from build123d import *

# Parameters (mm, degrees)
EXTRUDE_1_DEPTH     = 2
SKETCH_2_W          = 50
SKETCH_2_H          = 27
EXTRUDE_2_DEPTH     = 10
SKETCH_3_R          = 3
CUT_EXTRUDE_1_DEPTH = 13
SKETCH_5_W          = 47
SKETCH_5_H          = 1.6
CUT_EXTRUDE_2_DEPTH = 1.6
SKETCH_6_W          = 4
SKETCH_6_H          = 10
CUT_EXTRUDE_3_DEPTH = 7
SKETCH_7_W          = 80
SKETCH_7_H          = 14.002207555
CUT_EXTRUDE_4_DEPTH = 10
CUT_EXTRUDE_5_REACH = 14


with BuildPart() as part:
    # 草图1 → 凸台-拉伸1 (new body)
    with BuildSketch(Plane.XY):
        with BuildLine():
            Line((-46, 22.841953517), (-46, -22.841953517))
            Line((-46, -22.841953517), (-51, -31.502207555))
            Line((-51, -31.502207555), (-51, -39.502207555))
            ThreePointArc((-51, -39.502207555), (-46, -44.502207555), (-41, -39.502207555))
            Line((-41, -39.502207555), (-41, -31.502207555))
            Line((-41, -31.502207555), (36, -31.502207555))
            Line((36, -31.502207555), (36, -39.502207555))
            ThreePointArc((36, -39.502207555), (41, -44.502207555), (46, -39.502207555))
            Line((46, -39.502207555), (46, 39.502207555))
            ThreePointArc((46, 39.502207555), (41, 44.502207555), (36, 39.502207555))
            Line((36, 39.502207555), (36, 31.502207555))
            Line((36, 31.502207555), (-41, 31.502207555))
            Line((-41, 31.502207555), (-41, 39.502207555))
            ThreePointArc((-41, 39.502207555), (-46, 44.502207555), (-51, 39.502207555))
            Line((-51, 39.502207555), (-51, 31.502207555))
            Line((-51, 31.502207555), (-46, 22.841953517))
        make_face()
    extrude(amount=EXTRUDE_1_DEPTH)

    # 草图2 → 凸台-拉伸2 (add)
    with BuildSketch(Plane(origin=(0, 0, 0), x_dir=(-1, 0, 0), z_dir=(0, 0, -1))):
        with BuildLine():
            Line((46, -22.841953517), (46, 22.841953517))
            Line((46, 22.841953517), (51, 31.502207555))
            Line((51, 31.502207555), (51, 39.502207555))
            ThreePointArc((51, 39.502207555), (46, 44.502207555), (41, 39.502207555))
            Line((41, 39.502207555), (41, 31.502207555))
            Line((41, 31.502207555), (-36, 31.502207555))
            Line((-36, 31.502207555), (-36, 39.502207555))
            ThreePointArc((-36, 39.502207555), (-41, 44.502207555), (-46, 39.502207555))
            Line((-46, 39.502207555), (-46, -39.502207555))
            ThreePointArc((-46, -39.502207555), (-41, -44.502207555), (-36, -39.502207555))
            Line((-36, -39.502207555), (-36, -31.502207555))
            Line((-36, -31.502207555), (41, -31.502207555))
            Line((41, -31.502207555), (41, -39.502207555))
            ThreePointArc((41, -39.502207555), (46, -44.502207555), (51, -39.502207555))
            Line((51, -39.502207555), (51, -31.502207555))
            Line((51, -31.502207555), (46, -22.841953517))
        make_face()
        with Locations((-15, 0)):
            Rectangle(SKETCH_2_W, SKETCH_2_H, mode=Mode.SUBTRACT)
    extrude(amount=EXTRUDE_2_DEPTH)

    # 草图3 → 切除-拉伸1 (cut, through all)
    with BuildSketch(Plane(origin=(0, 0, -10), x_dir=(-1, 0, 0), z_dir=(0, 0, -1))):
        with Locations((-41, 39.502207555)):
            Circle(SKETCH_3_R)
        with Locations((46, -39.502207555)):
            Circle(SKETCH_3_R)
        with Locations((46, 39.502207555)):
            Circle(SKETCH_3_R)
        with Locations((-41, -39.502207555)):
            Circle(SKETCH_3_R)
    extrude(amount=-CUT_EXTRUDE_1_DEPTH, mode=Mode.SUBTRACT)

    # 草图5 → 切除-拉伸2 (cut)
    with BuildSketch(Plane(origin=(0, 0, 0), x_dir=(-1, 0, 0), z_dir=(0, 0, -1))):
        with Locations((-15.3, 10.95)):
            Rectangle(SKETCH_5_W, SKETCH_5_H)
        with Locations((-15.3, -10.95)):
            Rectangle(SKETCH_5_W, SKETCH_5_H)
    extrude(amount=-CUT_EXTRUDE_2_DEPTH, mode=Mode.SUBTRACT)

    # 草图6 → 切除-拉伸3 (cut, through all)
    with BuildSketch(Plane.ZY.offset(-40)):
        with Locations((-8, 0.5)):
            Rectangle(SKETCH_6_W, SKETCH_6_H)
    extrude(amount=-CUT_EXTRUDE_3_DEPTH, mode=Mode.SUBTRACT)

    # 草图7 → 切除-拉伸4 (cut)
    with BuildSketch(Plane(origin=(0, 0, -10), x_dir=(-1, 0, 0), z_dir=(0, 0, -1))):
        with Locations((4, -22.501103778)):
            Rectangle(SKETCH_7_W, SKETCH_7_H)
        Polygon((12, -15.5), (44, -15.5), (44, 29.502207555), (-36, 29.502207555), (-36, 15.5), (12, 15.5), align=None)
    extrude(amount=-CUT_EXTRUDE_4_DEPTH, mode=Mode.SUBTRACT)

    # 草图9 → 切除-拉伸5 (cut, up to next)
    with BuildSketch(Plane(origin=(0, 0, -10), x_dir=(-1, 0, 0), z_dir=(0, 0, -1)), mode=Mode.PRIVATE) as cut_extrude_5_sk1:
        Polygon((-46, -35.502207555), (-41.2, -28.502207555), (-41.2, 28.502207555), (-46, 35.502207555), align=None)
    cut_extrude_5_tool1 = extrude(cut_extrude_5_sk1.sketch, amount=-CUT_EXTRUDE_5_REACH, mode=Mode.PRIVATE) & part.part
    add(cut_extrude_5_tool1.solids().sort_by_distance((43.687494, 0, -10))[0], mode=Mode.SUBTRACT)


solid = part.part
Build history of the part. All positions in model axes, mm. A direction names the side the tool comes from. Round coordinates to 2 decimals unless told otherwise and drop trailing zeros. Loops run counter-clockwise (first coordinate to the right, second up) from the corner with the lowest first, then second, coordinate; pieces in that order, holes last. Notation, with made-up numbers: (83, 31) -> (139, 31) arc R32 ccw to (139, 58) -> close; hole circle Ø11 at (13, 4.25). An arc over 180 degrees is marked (long way). Use CSV: the item, a comma, the result in double quotes. Start each with the question number.
Q1. Flat gauge pins, fed straight in: pin 1 Ø3 at (x, z) = (13.5, -6) entering from -Y; pin 2 Ø2 at (x, y) = (28, 0) entering from -Z; pin 3 Ø5 at (y, z) = (-0.5, -6) entering from +X; pin 4 Ø5 at (x, y) = (41, 39.5) entering from +Z. Where does each tip first touch, or does it go through?
Q2. Mould opens along X. For faces 5 (the face through (-46, 0, -4)), 6 (the face through (43.634, -32.051, -4.084)), 7 (the face through (36, 23, -5)), 8 (the face through (-12, 0, -5)) say: +X half, -X half, draft (parallel to the pull), parting line (faces both ways), or undercut.
Q3. Saw through at C-C on z = -8.5. Count the separate pieces of the cut face and the enclosed holes in it, and give its area (3 significant figures).
Q4. Saw through at B-B on x = -20.5. Give the cut face in (y, z), and give its area (3 significant figures).
Q5. Drill centre lines: L1, parallel to Y at x = 41, z = -6.5; L2, parallel to Y at x = -5, z = -3; L3, parallel to X at y = -6.5, z = -3.5. Where is each one in solid material? Low to high.
Q6. Saw through at A-A on y = -21.5. Give the cut face in (x, z).
Q7. Which spindle directions (+Z, -Z, +X, -X, +Y, -Y) get a long thin tool onto all of the face, cutting with end or side? Do faces 1 (the face through (-41, -35, -4)), 2 (the face through (40, 0, -5)), 3 (the face through (43.6, 32, -4.1)), 4 (the face through (36, 35, -4)). Say none if no direction does.
Solutions:
1,pin 1,"stops at y = -31.5"
1,pin 2,"stops at z = 0"
1,pin 3,"stops at x = 41.2"
1,pin 4,"passes through"
2,face 5,"-X half"
2,face 6,"+X half"
2,face 7,"undercut"
2,face 8,"undercut"
3,separate pieces,"1"
3,enclosed holes,"5"
3,area,"1,300 mm^2"
4,outline,"(-31.5, -10) -> (-29.5, -10) -> (-29.5, 0) -> (29.5, 0) -> (29.5, -10) -> (31.5, -10) -> (31.5, 2) -> (-31.5, 2) -> close"
4,area,"166 mm^2"
5,L1,"y = -44.5 to -42.5, -36.5 to -4.5, 5.5 to 36.5, 42.5 to 44.5"
5,L2,"y = -31.5 to -29.5, -15.5 to -13.5, 13.5 to 15.5, 29.5 to 31.5"
5,L3,"x = -46 to -44, -12 to -10, 40 to 41.2"
6,outline,"(-46, -10) -> (-44, -10) -> (-44, 0) -> (36, 0) -> (36, -10) -> (41.2, -10) -> (41.2, 2) -> (-46, 2) -> close"
7,face 1,"+Z, -Z, -Y"
7,face 2,"-Z"
7,face 3,"+Z, -Z, +X"
7,face 4,"+Z, -Z, +Y"
